```python
from build123d import *

# Parameters (mm, degrees)
EXTRUDE_1_DEPTH     = 15
SKETCH_2_R          = 1.6
SKETCH_2_R_2        = 6.25
CUT_EXTRUDE_1_DEPTH = 2
SKETCH_3_R          = 1.35
CUT_EXTRUDE_2_DEPTH = 37
FILLET_1_R          = 2
FILLET_2_R          = 1
FILLET_3_R          = 3


with BuildPart() as part:
    # 草图1 → 凸台-拉伸1 (new, symmetric)
    with BuildSketch(Plane(origin=(0, 0, 0), x_dir=(1, 0, 0), z_dir=(0, 1, 0))):
        Polygon((0, 0), (0, 25.248427125), (-7.501572875, 32.75), (-40, 32.75), (-40, 30.75), (-8.33, 30.75), (-2, 24.42), (-2, 0), (-2, -24.42), (-8.33, -30.75), (-40, -30.75), (-40, -32.75), (-7.501572875, -32.75), (0, -25.248427125), align=None)
    extrude(amount=EXTRUDE_1_DEPTH, both=True)

    # 草图2 → 切除-拉伸1 (cut)
    with BuildSketch(Plane.ZY.offset(2)):
        with Locations((-20, 10.5)):
            Circle(SKETCH_2_R)
        with Locations((-8.5, 8.5)):
            Circle(SKETCH_2_R)
        with Locations((8.5, 8.5)):
            Circle(SKETCH_2_R)
        with Locations((20, 10.5)):
            Circle(SKETCH_2_R)
        with Locations((20, -10.5)):
            Circle(SKETCH_2_R)
        with Locations((8.5, -8.5)):
            Circle(SKETCH_2_R)
        with Locations((-8.5, -8.5)):
            Circle(SKETCH_2_R)
        with Locations((-20, -10.5)):
            Circle(SKETCH_2_R)
        Circle(SKETCH_2_R_2)
    extrude(amount=-CUT_EXTRUDE_1_DEPTH, mode=Mode.SUBTRACT)

    # 草图3 → 切除-拉伸2 (cut, symmetric)
    with BuildSketch(Plane.XY):
        with Locations((-23, 0)):
            Circle(SKETCH_3_R)
        with Locations((-26.514718626, -8.485281374)):
            Circle(SKETCH_3_R)
        with Locations((-35, -12)):
            Circle(SKETCH_3_R)
        with Locations((-35, 12)):
            Circle(SKETCH_3_R)
        with Locations((-26.514718626, 8.485281374)):
            Circle(SKETCH_3_R)
        with BuildLine():
            Line((-35, 6.25), (-40, 6.25))
            Line((-40, 6.25), (-40, -6.25))
            Line((-40, -6.25), (-35, -6.25))
            ThreePointArc((-35, -6.25), (-28.75, 0), (-35, 6.25))
        make_face()
    extrude(amount=CUT_EXTRUDE_2_DEPTH, both=True, mode=Mode.SUBTRACT)

    # 圆角1
    fillet_1_edges = [part.edges().sort_by_distance(p)[0] for p in [
        (-40, -6.25, -31.75),
        (-40, -6.25, 31.75),
        (-40, 6.25, -31.75),
        (-40, 6.25, 31.75),
        (-40, -15, 31.75),
        (-40, -15, -31.75),
        (-40, 15, -31.75),
        (-40, 15, 31.75),
    ]]
    fillet(fillet_1_edges, radius=FILLET_1_R)

    # 圆角2
    fillet_2_edges = [part.edges().sort_by_distance(p)[0] for p in [
        (-8.33, 0, 30.75),
        (-2, 0, 24.42),
        (-2, 0, -24.42),
        (-8.33, 0, -30.75),
    ]]
    fillet(fillet_2_edges, radius=FILLET_2_R)

    # 圆角3
    fillet_3_edges = [part.edges().sort_by_distance(p)[0] for p in [
        (0, 0, 25.248427125),
        (-7.501572875, 0, 32.75),
        (-7.501572875, 0, -32.75),
        (0, 0, -25.248427125),
    ]]
    fillet(fillet_3_edges, radius=FILLET_3_R)


solid = part.part
```
The listing builds one solid part. Answer for the finished solid, in the listing's coordinates (mm). A direction names the side the tool comes from. Give positions to 0.01 mm unless a question says otherwise; leave off trailing zeros. Write each loop counter-clockwise with the first axis right and the second up, starting at its lowest first coordinate (ties: lowest second). Pieces come first, ordered by that corner, then holes. Notation, with made-up numbers: (-7.75, -9.5) -> (43.25, -9.5) arc R19 cw to (43.25, 0.5) -> close; hole circle Ø6 at (83, -22). An arc over 180 degrees is marked (long way). Use one line per item in the form item = value.
1) Section A-A on x = -23 is taken. Write down the section's boundary in (y, z).
Result:
outline = (-15, -32.75) -> (-1.35, -32.75) -> (-1.35, -30.75) -> (-15, -30.75) -> close; (-15, 30.75) -> (-1.35, 30.75) -> (-1.35, 32.75) -> (-15, 32.75) -> close; (1.35, -32.75) -> (15, -32.75) -> (15, -30.75) -> (1.35, -30.75) -> close; (1.35, 30.75) -> (15, 30.75) -> (15, 32.75) -> (1.35, 32.75) -> close
2) Section C-C on y = 0 is taken. Count the separate pieces of the cut face and the enclosed holes in it, plus the area to 3 significant figures.
Result:
separate_pieces = 4
enclosed_holes = 0
area = 185 mm²
3) Straight lines are drawn through the part: probe 1 along Y at (x, z) = (-35, -31); probe 2 along Z at (x, y) = (-9.5, -4); probe 3 along X at (y, z) = (4.25, -18). For each, find the intervals that lie inside material, in ascending order.
Result:
probe_1 = -15 to -13.35, -10.65 to -6.25, 6.25 to 10.65, 13.35 to 15
probe_2 = -32.75 to -30.75, 30.75 to 32.75
probe_3 = -2 to 0
4) Section D-D on z = -20 is taken. Write down the section's boundary in (x, y).
Result:
outline = (-2, -15) -> (0, -15) -> (0, -12.1) -> (-2, -12.1) -> close; (-2, -8.9) -> (0, -8.9) -> (0, 8.9) -> (-2, 8.9) -> close; (-2, 12.1) -> (0, 12.1) -> (0, 15) -> (-2, 15) -> close
5) Section B-B on x = -13 is taken. Write down the section's boundary in (y, z).
Result:
outline = (-15, -32.75) -> (15, -32.75) -> (15, -30.75) -> (-15, -30.75) -> close; (-15, 30.75) -> (15, 30.75) -> (15, 32.75) -> (-15, 32.75) -> close
6) For a pull along Y with two mould halves and no side action, classify faces 4 (the cylindrical face through (-39.4, -14.43, -31.74)), 5 (the cylindrical face through (-27.586, 7.664, -31.736)), 6 (the cylindrical face through (-7.581, -0.21, 32.515)) as +Y half, -Y half, draft (parallel to the pull), parting line (faces both ways), or undercut.
Result:
face_4 = -Y half
face_5 = undercut
face_6 = draft
7) A tool of negligible diameter and unlimited length cuts with its end or side. For faces 1 (the flat face through (-5.12, 0.21, 27.54)), 2 (the flat face through (-1, -15, 0)), 3 (the flat face through (-36, 6.25, 32)), from which of +Z, -Z, +X, -X, +Y, -Y can it reach the whole face along a straight path? Write none if from no direction.
Result:
face_1 = -X, +Y, -Y
face_2 = +Z, -Z, +X, -X, -Y
face_3 = +Z, -Z, -X
8) Each of these flat-tipped pins is pushed along its axis until it touches: P1, Ø5, axis at y = 8.5, z = 8.5, coming from the -X side; P2, Ø4, axis at x = -5.5, y = -4.5, coming from the +Z side. Where does it stop, or does it pass through?
Result:
P1 = -2
P2 = 32.48
